```python
from build123d import *

# Parameters (mm, degrees)
SKETCH_1_R      = 8
SKETCH_1_R_2    = 4
EXTRUDE_1_DEPTH = 6
FILLET_1_R      = 10


with BuildPart() as part:
    # 草图1 → 凸台-拉伸1 (new body)
    # profile 1 of 3: a face of its own
    with BuildSketch(Plane.XY):
        with BuildLine():
            ThreePointArc((3, -7.416198487), (0, -8), (-3, -7.416198487))
            Line((-3, -7.416198487), (-3, -77.683801513))
            ThreePointArc((-3, -77.683801513), (0, -77.1), (3, -77.683801513))
            Line((3, -77.683801513), (3, -7.416198487))
        make_face()
        with BuildLine():
            ThreePointArc((-1.05, -55.1), (0, -54.05), (1.05, -55.1))
            Line((1.05, -55.1), (1.05, -70.1))
            ThreePointArc((1.05, -70.1), (0, -71.15), (-1.05, -70.1))
            Line((-1.05, -70.1), (-1.05, -55.1))
        make_face(mode=Mode.SUBTRACT)
        with BuildLine():
            ThreePointArc((-1.05, -37.5), (0, -36.45), (1.05, -37.5))
            Line((1.05, -37.5), (1.05, -45.1))
            ThreePointArc((1.05, -45.1), (0, -46.15), (-1.05, -45.1))
            Line((-1.05, -45.1), (-1.05, -37.5))
        make_face(mode=Mode.SUBTRACT)
        with BuildLine():
            ThreePointArc((-1.05, -12.5), (0, -11.45), (1.05, -12.5))
            Line((1.05, -12.5), (1.05, -27.5))
            ThreePointArc((1.05, -27.5), (0, -28.55), (-1.05, -27.5))
            Line((-1.05, -27.5), (-1.05, -12.5))
        make_face(mode=Mode.SUBTRACT)
    # profile 2 of 3: a face of its own
    with BuildSketch(Plane.XY):
        Circle(SKETCH_1_R)
        Circle(SKETCH_1_R_2, mode=Mode.SUBTRACT)
    # profile 3 of 3: a face of its own
    with BuildSketch(Plane.XY):
        with Locations((0, -85.1)):
            Circle(SKETCH_1_R)
        with Locations((0, -85.1)):
            Circle(SKETCH_1_R_2, mode=Mode.SUBTRACT)
    extrude(amount=EXTRUDE_1_DEPTH)

    # 圆角1
    fillet_1_edges = [part.edges().sort_by_distance(p)[0] for p in [
        (3, -77.683801513, 3),
        (-3, -77.683801513, 3),
        (-3, -7.416198487, 3),
        (3, -7.416198487, 3),
    ]]
    fillet(fillet_1_edges, radius=FILLET_1_R)


solid = part.part
```
Input: part model. Units: mm. Frame: model coordinates. A direction names the side the tool comes from. Give positions to 0.01 mm unless a question says otherwise; leave off trailing zeros. Loops run counter-clockwise (first coordinate to the right, second up) from the corner with the lowest first, then second, coordinate; pieces in that order, holes last. Notation, with made-up numbers: M -18.75,17.5 L -1.75,17.5 A16 cw -1.75,28.5 Z; hole C 12.5,44 d3. An arc over 180 degrees is marked long. Answer as CSV lines item,"result". Start each with the question number.
1. Section A-A on y = -59.5. Return loops of the section in (x, z).
2. Pull-direction query (X, two-part tool) for faces 3 (the face through (0, 8, 3)), 4 (the face through (1.05, -62, 3)), 5 (the face through (-3.74, -76.43, 3.04)), 6 (the face through (3.74, -76.43, 3.04)); classes: released by +X, released by -X, zero draft, split by the parting line, or undercut.
3. Section C-C on z = 1.8. Return loops of the section in (x, y).
4. Section D-D on y = 0. Return loops of the section in (x, z).
5. Section B-B on x = 0. Return loops of the section in (y, z).
6. Line query: L1, parallel to Y at x = 0, z = 4.3; L2, parallel to X at y = -85.5, z = 4.35; L3, parallel to Y at x = -0.5, z = 5.45. Output: solid intervals per line, ascending.
7. Reachability of faces 1 (the face through (0.02, -46.15, 2.96)), 2 (the face through (3, -43, 3)) from +Z, -Z, +X, -X, +Y, -Y: full face, straight path, thin tool, end or side. Return the list, or none.
8. Pin query (flat end, axial travel): P1, Ø3, axis at y = -40, z = 4, coming from the -X side; P2, Ø5, axis at x = -1.5, y = -19.5, coming from the -Z side; P3, Ø3, axis at y = -22.5, z = 4, coming from the +X side; P4, Ø5, axis at x = 0, y = 0, coming from the +Z side. Return the tip coordinate at first contact, or that it passes through.
Computed values:
1,outline,"M -3,0 L -1.05,0 L -1.05,6 L -3,6 Z; M 1.05,0 L 3,0 L 3,6 L 1.05,6 Z"
2,face 3,"split by the parting line"
2,face 4,"undercut"
2,face 5,"released by -X"
2,face 6,"released by +X"
3,outline,"M -5.78,-79.57 A8 ccw long 5.78,-79.57 A10 cw 3,-72.65 L 3,-12.45 A10 cw 5.78,-5.53 A8 ccw long -5.78,-5.53 A10 cw -3,-12.45 L -3,-72.65 A10 cw Z; hole C 0,-85.1 d8; hole C 0,0 d8; hole M -1.05,-70.1 A1.05 ccw 1.05,-70.1 L 1.05,-55.1 A1.05 ccw -1.05,-55.1 Z; hole M -1.05,-45.1 A1.05 ccw 1.05,-45.1 L 1.05,-37.5 A1.05 ccw -1.05,-37.5 Z; hole M -1.05,-27.5 A1.05 ccw 1.05,-27.5 L 1.05,-12.5 A1.05 ccw -1.05,-12.5 Z"
4,outline,"M -8,0 L -4,0 L -4,6 L -8,6 Z; M 4,0 L 8,0 L 8,6 L 4,6 Z"
5,outline,"M -93.1,0 L -89.1,0 L -89.1,6 L -93.1,6 Z; M -81.1,0 L -71.15,0 L -71.15,6 L -81.1,6 Z; M -54.05,0 L -46.15,0 L -46.15,6 L -54.05,6 Z; M -36.45,0 L -28.55,0 L -28.55,6 L -36.45,6 Z; M -11.45,0 L -4,0 L -4,6 L -11.45,6 Z; M 4,0 L 8,0 L 8,6 L 4,6 Z"
6,L1,"y = -93.1 to -89.1, -81.1 to -71.15, -54.05 to -46.15, -36.45 to -28.55, -11.45 to -4, 4 to 8"
6,L2,"x = -7.99 to -3.98, 3.98 to 7.99"
6,L3,"y = -93.08 to -89.07, -81.13 to -71.02, -54.18 to -46.02, -36.58 to -28.42, -11.58 to -3.97, 3.97 to 7.98"
7,face 1,"+Z, -Z"
7,face 2,"+Z, -Z, +X"
8,P1,"stops at x = -3"
8,P2,"stops at z = 0"
8,P3,"stops at x = 3"
8,P4,"passes through"
